Solid Edge part; units mm, degrees
sketch "Sketch1" plane through (0, 0, 0) normal (0, -1, 0) x (1, 0, 0)
  line L0 (-22.5, -72.5) -> (22.5, -72.5)
  line L1 (22.5, -72.5) -> (22.5, 72.5)
  line L2 (22.5, 72.5) -> (-22.5, 72.5)
  line L3 (-22.5, 72.5) -> (-22.5, -72.5)
extrude "Protrusion1" add sketch "Sketch1" against normal blind 2370
sketch "Sketch2" plane through (22.5, 1185, 0) normal (1, 0, 0) x (0, 1, 0)
  line L0 (1035, 72.5) -> (1035, 36.25)
  line L1 (1035, 36.25) -> (990, 36.25)
  line L2 (990, 36.25) -> (990, 72.5)
  line L3 (990, 72.5) -> (1035, 72.5)
  line L4 (-1035, 72.5) -> (-1035, 36.25)
  line L5 (-1035, 36.25) -> (-990, 36.25)
  line L6 (-990, 36.25) -> (-990, 72.5)
  line L7 (-990, 72.5) -> (-1035, 72.5)
extrude "ExtrudedCutout_1" cut sketch "Sketch2" against normal blind 89.2118
sketch "Sketch3" plane through (22.5, 1185, 0) normal (1, 0, 0) x (0, 1, 0)
  line L0 (-1185, -72.5) -> (1185, -72.5)
  line L1 (1185, -72.5) -> (1185, 0)
  line L2 (1185, 0) -> (-1185, 0)
  line L3 (-1185, 0) -> (-1185, -72.5)
extrude "ExtrudedCutout_2" cut sketch "Sketch3" against normal blind 236.7564
sketch "Sketch4" plane through (0, 1185, 0) normal (0, 0, -1) x (0, -1, 0)
  line L0 (-1185, 22.5) -> (1185, 22.5)
  line L1 (1185, 22.5) -> (1185, -22.5)
  line L2 (1185, -22.5) -> (-1185, -22.5)
  line L3 (-1185, -22.5) -> (-1185, 22.5)
extrude "ExtrudedProtrusion_2" add sketch "Sketch4" along normal blind 25
sketch "Sketch5" plane through (-22.5, 1185, 23.75) normal (-1, 0, 0) x (0, 1, 0)
  line L0 (-1185, -287.7315) -> (-1185, 76.8245)
  line L1 (-1185, 76.8245) -> (1185, 76.8245)
  line L2 (1185, 76.8245) -> (1185, 51.6762)
  line L3 (1185, 51.6762) -> (-1185, -287.7315)
extrude "ExtrudedCutout_5" cut sketch "Sketch5" against normal blind 75.1515
properties material "Wood, Pine"
Work out the finished part from the listing and answer in its coordinate system (mm). A direction names the side the tool comes from. Give positions to 0.01 mm unless a question says otherwise; leave off trailing zeros. Order: outer loops, then holes, each group sorted by start corner. A loop starts at its lowest first (then second) coordinate and runs counter-clockwise, first axis right, second up. Notation, with made-up numbers: (24.5, 55) - (54.5, 55) arc R20 ccw to (54.5, 83) - close; hole circle Ø1 at (24.25, 32). An arc over 180 degrees is marked (long way). One line per item, written item: value. Start each with the question number.
1. Each of these flat-tipped pins is pushed along its axis until it touches: pin 1 Ø2 at (x, y) = (15, 1884) entering from -Z; pin 2 Ø8 at (x, y) = (16.5, 2020) entering from -Z; pin 3 Ø22.5 at (x, y) = (-5.5, 2189.5) entering from +Z. Where does it stop, or does it pass through?
2. Which of the six approach directions +Z, -Z, +X, -X, +Y, -Y give full straight-line access (tool end or side, diameter ignored) to faces 4 (the face through (0, 2294, 72.5)), 5 (the face through (0, 2198, 36.25))?
3. Section C-C, the plane y = 1836.5 is taken. Write down the section's boundary in (x, z).
4. Section B-B, the plane x = -9 is taken. Write down the section's boundary in (y, z).
5. For a pull along Y with two mould halves and no side action, classify faces 1 (the face through (0, 2175, 54)), 2 (the face through (0, 2370, 24)), 3 (the face through (-22.5, 2092, 35)) as released by +Y, released by -Y, zero draft, split by the parting line, or undercut.
6. Section A-A, the plane z = 48 is taken. Write down the section's boundary in (x, y), then the cut area to 3 significant figures.
7. Section D-D, the plane z = -8.5 is taken. Write down the section's boundary in (x, y).
8. Consider line 1 (Z direction, x = 14, y = 1890); line 2 (Z direction, x = -12, y = 1905). Determine where each line is inside the solid, lowest interval first.
Filled sheet:
1. pin 1: z = 41.53
1. pin 2: z = 21.62
1. pin 3: z = 36.25
2. face 4: +Z, +X, -X, +Y, -Y
2. face 5: +Z, +X, -X
3. outline: (-22.5, 48.48) - (22.5, 48.48) - (22.5, 72.5) - (-22.5, 72.5) - close
4. outline: (1668.75, 72.5) - (2349.57, -25) - (2370, -25) - (2370, 72.5) - (2220, 72.5) - (2220, 36.25) - (2175, 36.25) - (2175, 72.5) - close
5. face 1: undercut
5. face 2: released by +Y
5. face 3: zero draft
6. outline: (-22.5, 1839.83) - (22.5, 1839.83) - (22.5, 2175) - (-22.5, 2175) - close; (-22.5, 2220) - (22.5, 2220) - (22.5, 2370) - (-22.5, 2370) - close
6. area: 21,800 mm²
7. outline: (-22.5, 2234.35) - (22.5, 2234.35) - (22.5, 2370) - (-22.5, 2370) - close
8. line 1: 40.81 to 72.5
8. line 2: 38.67 to 72.5
